Build history of the part. All positions in model axes, mm. Face numbers are marked on the shaded views. A direction names the side the tool comes from. Coordinates: 2 decimals unless noted, no trailing zeros. Order: outer loops, then holes, each group sorted by start corner. A loop starts at its lowest first (then second) coordinate and runs counter-clockwise, first axis right, second up. Notation, with made-up numbers: M -9.75,-23.75 L 9.25,-23.75 A24 cw 9.25,1.25 Z; hole C -34.75,38.25 d3. An arc over 180 degrees is marked long. Write item = value, one per line. Start each with the question number.
Q1. Band-saw the part on B-B on x = 7.5. Write the cut outline in (y, z) (1 decimal), plus the area to 3 significant figures.
Q2. 3-axis set-ups, long thin cutter, end or side, ignore diameter. For the marked faces 1 and 2: which of +Z, -Z, +X, -X, +Y, -Y reach the whole face in a straight line?
Q3. Pin check, flat tip, straight feed: P1, Ø1.7, axis at x = 24.5, z = -96.5, coming from the -Y side. Stop position of the tip, or through.
Q4. Band-saw the part on C-C on z = -2.5. Write the cut outline in (x, y).
Q5. Pull direction X, two halves, no side cores. Call the marked faces 3, 4 and 5: released by +X, released by -X, zero draft, split by the parting line, or undercut.
Q6. Band-saw the part on A-A on y = -6.35. Write the cut outline in (x, z) (1 decimal), plus the area to 3 significant figures.
Q7. Band-saw the part on D-D on z = -38.1. Write the cut outline in (x, y), plus the area to 3 significant figures.
Q8. Drill centre lines: probe 1 along Z at (x, y) = (0, 11.85) (1 decimal); probe 2 along Z at (x, y) = (-19.05, 12) (3 decimals); probe 3 along Y at (x, z) = (-10, 11). Where is each one in solid material? Low to high.
```python
from build123d import *

# Parameters (mm, degrees)
BOSS_EXTRUDE1_DEPTH      = 98.424999
BOSS_EXTRUDE1_DEPTH_BACK = 98.424999
SKETCH3_W                = 50.8
SKETCH3_H                = 25.4
SKETCH3_W_2              = 47.625
SKETCH3_H_2              = 22.225
SKETCH4_R                = 14.2875
CUT_EXTRUDE3_DEPTH       = 105.774999061
CUT_EXTRUDE5_DEPTH       = 1.5875
CUT_EXTRUDE6_DEPTH       = 1.5875
F_10_CLEARANCE_HOLE1_D   = 4.9784


with BuildPart() as part:
    # Sketch3 → Boss-Extrude1 (new, two sides: drawn at the far end of the back side and taken through both)
    with BuildSketch(Plane.XY.offset(-BOSS_EXTRUDE1_DEPTH_BACK)):
        Rectangle(SKETCH3_W, SKETCH3_H)
        Rectangle(SKETCH3_W_2, SKETCH3_H_2, mode=Mode.SUBTRACT)
    extrude(amount=BOSS_EXTRUDE1_DEPTH + BOSS_EXTRUDE1_DEPTH_BACK)

    # Sketch4 → Cut-Extrude3 (cut, through all)
    with BuildSketch(Plane.XZ.offset(12.7)):
        with Locations((0, 73.025)):
            Circle(SKETCH4_R)
        with Locations((0, -73.025)):
            Circle(SKETCH4_R)
    extrude(amount=-CUT_EXTRUDE3_DEPTH, mode=Mode.SUBTRACT)

    # Sketch5 → Cut-Extrude5 (cut)
    with BuildSketch(Plane(origin=(25.4, 0, 0), x_dir=(0, 0, -1), z_dir=(1, 0, 0))):
        with BuildLine():
            Line((98.424999492, 0), (98.424999492, -12.7))
            Line((98.424999492, -12.7), (95.249999492, -12.7))
            ThreePointArc((95.249999492, -12.7), (88.899999492, -6.35), (95.249999492, 0))
            Line((95.249999492, 0), (98.424999492, 0))
        make_face()
    extrude(amount=-CUT_EXTRUDE5_DEPTH, mode=Mode.SUBTRACT)

    # Sketch6 → Cut-Extrude6 (cut)
    with BuildSketch(Plane.XZ.offset(12.7)):
        Polygon((23.8125, -98.424999492), (23.8125, -95.249999492), (16.1925, -98.424999492), align=None)
    extrude(amount=-CUT_EXTRUDE6_DEPTH, mode=Mode.SUBTRACT)

    # #10 Clearance Hole1 (through all)
    with Locations(Plane(origin=(0, -12.7, 0), x_dir=(-1, 0, 0), z_dir=(0, -1, 0))):
        with Locations((-19.05, 85.724999492), (19.05, 92.074999492), (19.05, 38.099999492), (-19.05, 38.099999492)):
            Hole(F_10_CLEARANCE_HOLE1_D / 2)


solid = part.part
```
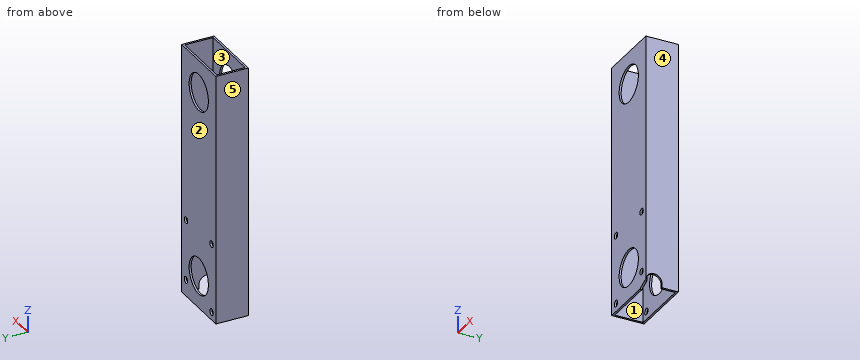
Recorded:
q1.outline = M -12.7,-98.4 L -11.1,-98.4 L -11.1,-85.2 L -12.7,-85.2 Z; M -12.7,-60.9 L -11.1,-60.9 L -11.1,60.9 L -12.7,60.9 Z; M -12.7,85.2 L -11.1,85.2 L -11.1,98.4 L -12.7,98.4 Z; M 11.1,-98.4 L 12.7,-98.4 L 12.7,-85.2 L 11.1,-85.2 Z; M 11.1,-60.9 L 12.7,-60.9 L 12.7,60.9 L 11.1,60.9 Z; M 11.1,85.2 L 12.7,85.2 L 12.7,98.4 L 11.1,98.4 Z
q1.area = 471 mm2
q2.face_1 = +Z, -Z
q2.face_2 = +Z, -Z, +X, -X, +Y
q3.P1 = 0
q4.outline = M -25.4,-12.7 L 25.4,-12.7 L 25.4,12.7 L -25.4,12.7 Z; hole M -23.81,-11.11 L 23.81,-11.11 L 23.81,11.11 L -23.81,11.11 Z
q5.face_3 = undercut
q5.face_4 = released by +X
q5.face_5 = released by -X
q6.outline = M -25.4,-98.4 L -23.8,-98.4 L -23.8,98.4 L -25.4,98.4 Z; M 23.8,-88.9 L 25.4,-88.9 L 25.4,98.4 L 23.8,98.4 Z
q6.area = 610 mm2
q7.outline = M -25.4,-12.7 L -21.54,-12.7 L -21.54,-11.11 L -23.81,-11.11 L -23.81,11.11 L -21.54,11.11 L -21.54,12.7 L -25.4,12.7 Z; M -16.56,-12.7 L 16.56,-12.7 L 16.56,-11.11 L -16.56,-11.11 Z; M -16.56,11.11 L 16.56,11.11 L 16.56,12.7 L -16.56,12.7 Z; M 21.54,-12.7 L 25.4,-12.7 L 25.4,12.7 L 21.54,12.7 L 21.54,11.11 L 23.81,11.11 L 23.81,-11.11 L 21.54,-11.11 Z
q7.area = 200 mm2
q8.probe_1 = -98.4 to -87.3, -58.7 to 58.7, 87.3 to 98.4
q8.probe_2 = -98.425 to -94.564, -89.586 to -40.589, -35.611 to 98.425
q8.probe_3 = -12.7 to -11.11, 11.11 to 12.7
